```python
from build123d import *

# Parameters (mm, degrees)
SKETCH_1_W           = 20
SKETCH_1_H           = 40
EXTRUDE_1_DEPTH      = 40
SKETCH_2_R           = 1
CUT_EXTRUDE_3_DEPTH  = 40
EXTRUDE_2_DEPTH      = 5
EXTRUDE_2_DEPTH_BACK = 45
SKETCH_4_R           = 1.5
CHAMFER_1_SIZE       = 2
FILLET_1_R           = 1
SKETCH_5_R           = 3
EXTRUDE_3_DEPTH      = 50
EXTRUDE_4_DEPTH      = 1.5
EXTRUDE_4_DEPTH_BACK = 53
SKETCH_7_R           = 3
SKETCH_12_W          = 1.5
SKETCH_12_H          = 6.856105301
CUT_EXTRUDE_6_DEPTH  = 25.5
EXTRUDE_START        = 6.5
SKETCH_9_R           = 3
EXTRUDE_7_DEPTH      = 6.5


with BuildPart() as part:
    # ｽｹｯﾁ1 → ﾎﾞｽ - 押し出し1 (new body)
    with BuildSketch(Plane(origin=(0, 0, 0), x_dir=(0, 0, -1), z_dir=(1, 0, 0))):
        with Locations((-16.51810585, 9.247910864)):
            Rectangle(SKETCH_1_W, SKETCH_1_H)
    extrude(amount=EXTRUDE_1_DEPTH)

    # ｽｹｯﾁ2 → ｶｯﾄ - 押し出し3 (cut)
    with BuildSketch(Plane.ZY):
        with Locations((9.01810585, 26.201539891)):
            Circle(SKETCH_2_R)
        with Locations((9.01810585, 11.201539891)):
            Circle(SKETCH_2_R)
        with Locations((24.01810585, 11.201539891)):
            Circle(SKETCH_2_R)
        with Locations(Location((24.01810585, 26.201539891, 0), (0, 0, 180))):
            Circle(SKETCH_2_R)
    extrude(amount=-CUT_EXTRUDE_3_DEPTH, mode=Mode.SUBTRACT)

    # ｽｹｯﾁ4 → ﾎﾞｽ - 押し出し2 (add, two sides: drawn at the far end of the back side and taken through both)
    with BuildSketch(Plane.ZY.offset(-EXTRUDE_2_DEPTH_BACK)):
        with Locations((16.51810585, -0.752089136)):
            Circle(SKETCH_4_R)
    extrude(amount=EXTRUDE_2_DEPTH + EXTRUDE_2_DEPTH_BACK)

    # 面取り1
    chamfer_1_edges = [part.edges().sort_by_distance(p)[0] for p in [
        (20, -10.752089136, 6.51810585),
        (20, -10.752089136, 26.51810585),
        (20, 29.247910864, 26.51810585),
        (20, 29.247910864, 6.51810585),
    ]]
    chamfer(chamfer_1_edges, length=CHAMFER_1_SIZE)

    # ﾌｨﾚｯﾄ1
    fillet_1_edges = [part.edges().sort_by_distance(p)[0] for p in [
        (0, 9.247910864, 26.51810585),
        (40, 9.247910864, 26.51810585),
        (0, 9.247910864, 6.51810585),
        (0, -10.752089136, 16.51810585),
        (0, 29.247910864, 16.51810585),
        (0, -9.752089136, 25.51810585),
        (0, -9.752089136, 7.51810585),
        (0, 28.247910864, 7.51810585),
        (0, 28.247910864, 25.51810585),
        (40, 29.247910864, 16.51810585),
        (40, 9.247910864, 6.51810585),
        (40, -10.752089136, 16.51810585),
        (40, -9.752089136, 25.51810585),
        (40, -9.752089136, 7.51810585),
        (40, 28.247910864, 7.51810585),
        (40, 28.247910864, 25.51810585),
    ]]
    fillet(fillet_1_edges, radius=FILLET_1_R)

    # ｽｹｯﾁ5 → ﾎﾞｽ - 押し出し3 (add)
    with BuildSketch(Plane.ZY.offset(5)):
        with Locations((16.51810585, -0.752089136)):
            Circle(SKETCH_5_R)
    extrude(amount=-EXTRUDE_3_DEPTH)

    # ｽｹｯﾁ7 → ﾎﾞｽ - 押し出し4 (add, two sides: drawn at the far end of the back side and taken through both)
    with BuildSketch(Plane.ZY.offset(5).offset(-EXTRUDE_4_DEPTH_BACK)):
        with Locations((16.51810585, -0.752089136)):
            Circle(SKETCH_7_R)
    extrude(amount=EXTRUDE_4_DEPTH + EXTRUDE_4_DEPTH_BACK)

    # ｽｹｯﾁ12 → ｶｯﾄ - 押し出し6 (cut)
    with BuildSketch(Plane.XY):
        with Locations((47.25, -0.324036486)):
            Rectangle(SKETCH_12_W, SKETCH_12_H)
    extrude(amount=CUT_EXTRUDE_6_DEPTH, mode=Mode.SUBTRACT)

    # ｽｹｯﾁ9 → ﾎﾞｽ - 押し出し7 (add)
    with BuildSketch(Plane.ZY.offset(EXTRUDE_START)):
        with Locations((16.51810585, -0.752089136)):
            Circle(SKETCH_9_R)
    extrude(amount=-EXTRUDE_7_DEPTH)


solid = part.part
```
Read the model definition and answer for the solid it produces. Units are mm, in the model's axes. A direction names the side the tool comes from. Give positions to 0.01 mm unless a question says otherwise; leave off trailing zeros. Order: outer loops, then holes, each group sorted by start corner. A loop starts at its lowest first (then second) coordinate and runs counter-clockwise, first axis right, second up.
(1) Given pin 1 (1.8 mm diameter, centred on y = 11.2, z = 9.02, fed in from -X); pin 2 (4 mm diameter, centred on y = 2, z = 21.5, fed in from +X); pin 3 (1.5 mm diameter, centred on x = 0, y = 3.5, fed in from -Z), each flat-ended and moving along its own axis, determine where each tip first touches the part or whether it passes through.
(2) For faces 4 (the flat face through (19.734, 28.262, 25.504)), 5 (the cylindrical face through (-3.2, -0.62, 13.52)), 6 (the cylindrical face through (43.3, -0.62, 13.52)), determine the directions among +Z, -Z, +X, -X, +Y, -Y from which every point of the face is accessible in a straight line to the end or side of a thin tool.
(3) Straight lines are drawn through the part: L1, parallel to Z at x = 2, y = 10.5; L2, parallel to Y at x = 39, z = 9.5; L3, parallel to X at y = 17.5, z = 18.5. For each, find the intervals that lie inside material, in ascending order.
(4) Find section B-B (z = 21.25). Give the vertices of the cut face in (x, y).
(5) Find section D-D (z = 15.5). Give the vertices of the cut face in (x, y), plus the area to 3 significant figures.
(6) For a pull along Z with two mould halves and no side action, classify faces 1 (the cylindrical face through (19.72, 12.193, 8.888)), 2 (the flat face through (20, -10.752, 17)), 3 (the flat face through (20, 9, 6.518)) as released by +Z, released by -Z, zero draft, split by the parting line, or undercut.
(7) Find section A-A (y = -7). Give the vertices of the cut face in (x, z), plus the area to 3 significant figures.
(8) Find section C-C (x = 2.5). Give the vertices of the cut face in (y, z).
Result sheet:
1. pin 1: passes through
1. pin 2: stops at x = 40
1. pin 3: stops at z = 6.55
2. face 4: +Z, +X, -X, +Y
2. face 5: -X
2. face 6: +X
3. L1: z = 6.52 to 8.31, 9.73 to 23.31, 24.73 to 26.52
3. L2: y = -10.75 to 10.33, 12.08 to 25.33, 27.08 to 29.25
3. L3: x = 0 to 40
4. outline: (0, -9.75) arc R1 ccw to (1, -10.75) - (39, -10.75) arc R1 ccw to (40, -9.75) - (40, 28.25) arc R1 ccw to (39, 29.25) - (1, 29.25) arc R1 ccw to (0, 28.25) - close
5. outline: (-6.5, -3.57) - (0, -3.57) - (0, -9.75) arc R1 ccw to (1, -10.75) - (39, -10.75) arc R1 ccw to (40, -9.75) - (40, -3.57) - (46.5, -3.57) - (46.5, 2.07) - (40, 2.07) - (40, 28.25) arc R1 ccw to (39, 29.25) - (1, 29.25) arc R1 ccw to (0, 28.25) - (0, 2.07) - (-6.5, 2.07) - close
5. area: 1,670 mm2
6. face 1: undercut
6. face 2: zero draft
6. face 3: released by -Z
7. outline: (0, 7.52) arc R1 ccw to (1, 6.52) - (39, 6.52) arc R1 ccw to (40, 7.52) - (40, 25.52) arc R1 ccw to (39, 26.52) - (1, 26.52) arc R1 ccw to (0, 25.52) - close
7. area: 799 mm2
8. outline: (-10.75, 8.52) - (-8.75, 6.52) - (27.25, 6.52) - (29.25, 8.52) - (29.25, 24.52) - (27.25, 26.52) - (-8.75, 26.52) - (-10.75, 24.52) - close; hole circle Ø2 at (11.2, 9.02); hole circle Ø2 at (11.2, 24.02); hole circle Ø2 at (26.2, 9.02); hole circle Ø2 at (26.2, 24.02)
